from build123d import *

# Parameters (mm, degrees)
SKETCH1_W           = 81
SKETCH1_H           = 100
BOSS_EXTRUDE1_DEPTH = 0.5
CUT_EXTRUDE1_DEPTH  = 65.352544627
M2_HOLE1_AD_D       = 2.4
M2_HOLE1_AD_DEPTH   = 100
M2_HOLE1_AD_TIP     = 0.721032743
M2_HOLE2_AD_D       = 2.4
M2_HOLE2_AD_DEPTH   = 100
M2_HOLE2_AD_TIP     = 0.721032743
M2_HOLE3_AE_D       = 2.4
M2_HOLE3_AE_DEPTH   = 200
M2_HOLE3_AE_TIP     = 0.721032743
FILLET1_R           = 0.1


with BuildPart() as part:
    # Sketch1 → Boss-Extrude1 (new, symmetric)
    with BuildSketch(Plane.XY):
        Rectangle(SKETCH1_W, SKETCH1_H)
    extrude(amount=BOSS_EXTRUDE1_DEPTH, both=True)

    # Sketch2 → Cut-Extrude1 (cut, through all)
    with BuildSketch(Plane.XY.offset(0.5)):
        with BuildLine():
            Line((-30, -38), (30, -38))
            ThreePointArc((30, -38), (33.535533906, -36.535533906), (35, -33))
            Line((35, -33), (35, 33))
            ThreePointArc((35, 33), (33.535533906, 36.535533906), (30, 38))
            Line((30, 38), (-30, 38))
            ThreePointArc((-30, 38), (-33.535533906, 36.535533906), (-35, 33))
            Line((-35, 33), (-35, -33))
            ThreePointArc((-35, -33), (-33.535533906, -36.535533906), (-30, -38))
        make_face()
    extrude(amount=-CUT_EXTRUDE1_DEPTH, mode=Mode.SUBTRACT)

    # M2 Hole1 - AD
    with Locations(Plane.XY.offset(0.5)):
        with Locations((-30.5, 40.5), (30.5, 40.5), (-30.5, -40.5), (30.5, -40.5)):
            Hole(M2_HOLE1_AD_D / 2, depth=M2_HOLE1_AD_DEPTH)
            with Locations((0, 0, -(M2_HOLE1_AD_DEPTH + M2_HOLE1_AD_TIP / 2))):  # 118° drill point
                Cone(0, M2_HOLE1_AD_D / 2, M2_HOLE1_AD_TIP, mode=Mode.SUBTRACT)

    # M2 Hole2 - AD
    with Locations(Plane.XY.offset(0.5)):
        with Locations((-21.5, 47.5), (21.5, 47.5), (-21.5, -47.5), (21.5, -47.5)):
            Hole(M2_HOLE2_AD_D / 2, depth=M2_HOLE2_AD_DEPTH)
            with Locations((0, 0, -(M2_HOLE2_AD_DEPTH + M2_HOLE2_AD_TIP / 2))):  # 118° drill point
                Cone(0, M2_HOLE2_AD_D / 2, M2_HOLE2_AD_TIP, mode=Mode.SUBTRACT)

    # M2 Hole3 - AE
    with Locations(Plane.XY.offset(0.5)):
        with Locations((0, 47.5), (0, -47.5)):
            Hole(M2_HOLE3_AE_D / 2, depth=M2_HOLE3_AE_DEPTH)
            with Locations((0, 0, -(M2_HOLE3_AE_DEPTH + M2_HOLE3_AE_TIP / 2))):  # 118° drill point
                Cone(0, M2_HOLE3_AE_D / 2, M2_HOLE3_AE_TIP, mode=Mode.SUBTRACT)

    # Fillet1
    fillet1_edges = [part.edges().sort_by_distance(p)[0] for p in [
        (-40.5, 0, 0.5),
        (40.5, 0, 0.5),
        (-40.5, 0, -0.5),
        (40.5, 0, -0.5),
    ]]
    fillet(fillet1_edges, radius=FILLET1_R)


solid = part.part
CAD build for the part. Positions are in the model's coordinates, mm. A direction names the side the tool comes from. Give positions to 0.01 mm unless a question says otherwise; leave off trailing zeros. Write each loop counter-clockwise with the first axis right and the second up, starting at its lowest first coordinate (ties: lowest second). Pieces come first, ordered by that corner, then holes. Notation, with made-up numbers: M -28,77 L -3,77 A18 ccw -3,99 Z; hole C 13.25,88 d11. An arc over 180 degrees is marked long. Put each result on its own line as item: value. Start each with the question number.
(1) Band-saw the part on B-B, the plane y = 26.5. Write the cut outline in (x, z).
(2) Band-saw the part on C-C, the plane z = 0.05. Give the number of separate pieces and of enclosed holes in the cut face, and give its area (3 significant figures).
(3) Probe L1, parallel to Y at x = 30.5, z = -0.25; L2, parallel to Y at x = 4.5, z = 0; L3, parallel to X at y = -1, z = -0.25. List the from-to ranges inside material, lowest first.
(4) Which spindle directions (+Z, -Z, +X, -X, +Y, -Y) get a long thin tool onto all of the face, cutting with end or side? Do faces 4 (the face through (-34, -36, 0)), 5 (the face through (-36, 1, 0.5)). Say none if no direction does.
(5) Band-saw the part on D-D, the plane x = 21.5. Write the cut outline in (y, z).
(6) Band-saw the part on A-A, the plane x = -8. Write the cut outline in (y, z), and give its area (3 significant figures).
(7) Mould opens along X. For faces 1 (the face through (-21.34, -46.31, -0.01)), 2 (the face through (29.85, 41.51, -0.01)), 3 (the face through (-36, 1, -0.5)) say: +X half, -X half, draft (parallel to the pull), parting line (faces both ways), or undercut.
Response values:
1. outline: M -40.5,-0.4 A0.1 ccw -40.4,-0.5 L -35,-0.5 L -35,0.5 L -40.4,0.5 A0.1 ccw -40.5,0.4 Z; M 35,-0.5 L 40.4,-0.5 A0.1 ccw 40.5,-0.4 L 40.5,0.4 A0.1 ccw 40.4,0.5 L 35,0.5 Z
2. separate pieces: 1
2. enclosed holes: 11
2. area: 2,760 mm2
3. L1: y = -50 to -41.7, -39.3 to -37.97, 37.97 to 39.3, 41.7 to 50
3. L2: y = -50 to -38, 38 to 50
3. L3: x = -40.5 to -35, 35 to 40.5
4. face 4: +Z, -Z
4. face 5: +Z, +X, -X, +Y, -Y
5. outline: M -50,-0.5 L -48.7,-0.5 L -48.7,0.5 L -50,0.5 Z; M -46.3,-0.5 L -38,-0.5 L -38,0.5 L -46.3,0.5 Z; M 38,-0.5 L 46.3,-0.5 L 46.3,0.5 L 38,0.5 Z; M 48.7,-0.5 L 50,-0.5 L 50,0.5 L 48.7,0.5 Z
6. outline: M -50,-0.5 L -38,-0.5 L -38,0.5 L -50,0.5 Z; M 38,-0.5 L 50,-0.5 L 50,0.5 L 38,0.5 Z
6. area: 24.0 mm2
7. face 1: undercut
7. face 2: undercut
7. face 3: draft
